from build123d import *

# Parameters (mm, degrees)
F0_R      = 19.05
F0_R_2    = 17.78
F0_R_3    = 9.525
F1_DEPTH  = 1.27
F2_DEPTH  = 151.13
F3_DEPTH  = 76.2
F5_DEPTH  = 25
F6_START  = -5.08
F6_DEPTH  = 3.302
F7_DEPTH  = 1
F8_DEPTH  = 1
F10_DEPTH = 25


with BuildPart() as f1:
    # F0 (on Top) → F1 (new body)
    with BuildSketch(Plane.XY):
        with Locations((-55.5866120592, 34.7886830568)):
            Circle(F0_R)
        with Locations((-55.5866120592, 34.7886830568)):
            Circle(F0_R_2, mode=Mode.SUBTRACT)
        with Locations((-55.5866120592, 34.7886830568)):
            Circle(F0_R_2)
        with Locations((-55.5866120592, 34.7886830568)):
            Circle(F0_R_3, mode=Mode.SUBTRACT)
        with BuildLine():
            ThreePointArc((4.7383879408, 34.7886830568), (-9.5491120592, 49.0761830568), (-23.8366120592, 34.7886830568))
            ThreePointArc((-23.8366120592, 34.7886830568), (-9.5491120592, 20.5011830568), (4.7383879408, 34.7886830568))
        make_face()
        Polygon((2.9366439238, 30.5109386121), (-7.0108694278, 21.8368289678), (-19.4966254107, 26.1145734125), (-22.0348680421, 39.0664275016), (-12.0873546906, 47.7405371459), (0.3984012923, 43.4627927011), align=None, mode=Mode.SUBTRACT)
        Polygon((-19.4966254107, 26.1145734125), (-7.0108694278, 21.8368289678), (2.9366439238, 30.5109386121), (0.3984012923, 43.4627927011), (-12.0873546906, 47.7405371459), (-22.0348680421, 39.0664275016), align=None)
    extrude(amount=-F1_DEPTH)

    # F0 (on Top) → F2 (join)
    with BuildSketch(Plane.XY):
        with Locations((-55.5866120592, 34.7886830568)):
            Circle(F0_R)
        with Locations((-55.5866120592, 34.7886830568)):
            Circle(F0_R_2, mode=Mode.SUBTRACT)
        with BuildLine():
            ThreePointArc((4.7383879408, 34.7886830568), (-9.5491120592, 49.0761830568), (-23.8366120592, 34.7886830568))
            ThreePointArc((-23.8366120592, 34.7886830568), (-9.5491120592, 20.5011830568), (4.7383879408, 34.7886830568))
        make_face()
        Polygon((2.9366439238, 30.5109386121), (-7.0108694278, 21.8368289678), (-19.4966254107, 26.1145734125), (-22.0348680421, 39.0664275016), (-12.0873546906, 47.7405371459), (0.3984012923, 43.4627927011), align=None, mode=Mode.SUBTRACT)
    extrude(amount=F2_DEPTH)



with BuildPart() as f3:
    # F0 (on Top) → F3 (new body)
    with BuildSketch(Plane.XY):
        Polygon((-36.5366120592, 53.8386830568), (-36.5366120592, 34.7886830568), (-36.5366120592, 15.7386830568), (-23.8366120592, 15.7386830568), (-23.8366120592, 34.7886830568), (-23.8366120592, 53.8386830568), align=None)
    extrude(amount=F3_DEPTH)

    # F4 (on face) → F5 (cut)
    with BuildSketch(Plane.YZ.offset(-23.8366120592)):
        Polygon((15.7386830568, 76.2), (53.8386830568, 44.2303040521), (53.8386830568, 76.2), align=None)
        Polygon((53.8386830568, 0), (53.8386830568, 9.1670642607), (15.7386830568, 41.1367602085), (15.7386830568, 0), align=None)
    extrude(amount=-F5_DEPTH, mode=Mode.SUBTRACT)

    # F4 (on face) → F6 (cut)
    with BuildSketch(Plane.YZ.offset(-23.8366120592).offset(F6_START)):
        Polygon((53.8386830568, 11.7778788393), (53.8386830568, 41.6194894735), (15.7386830568, 73.5891854213), (15.7386830568, 43.7475747872), align=None)
    extrude(amount=-F6_DEPTH, mode=Mode.SUBTRACT)


with BuildPart() as f1_1:
    add(f1.part)
    # F7 (add): a face of the model
    f7_faces = [f3.part.faces().sort_by_distance(p)[0] for p in [
        (-36.5366120592, 34.7886830568, 42.6835321303),
    ]]

    add(f3.part)  # F7 merges F3
    extrude(f7_faces, amount=F7_DEPTH)

    # F8 (add): faces of the model
    f8_faces = [f1_1.faces().sort_by_distance(p)[0] for p in [
        (-23.8366120592, 25.2636830568, 50.6759561173),
        (-23.8366120592, 44.3136830568, 34.6911081434),
    ]]
    extrude(f8_faces, amount=F8_DEPTH)

    # F9 (on face) → F10 (cut)
    with BuildSketch(Plane(origin=(0, 0, -1.27), x_dir=(1, 0, 0), z_dir=(0, 0, -1))):
        Polygon((-12.0873546906, -47.7405371459), (-5.8444766991, -45.6016649235), (-17.0611113664, -43.4034823237), align=None)
    extrude(amount=-F10_DEPTH, mode=Mode.SUBTRACT)


solid = f1_1.part
CAD build for the part. Positions are in the model's coordinates, mm. A direction names the side the tool comes from. Coordinates: 2 decimals unless noted, no trailing zeros. Order: outer loops, then holes, each group sorted by start corner. A loop starts at its lowest first (then second) coordinate and runs counter-clockwise, first axis right, second up. Notation, with made-up numbers: (70, 82.25) -> (82, 82.25) arc R24 ccw to (82, 109.25) -> close; hole circle Ø8 at (47, 39). An arc over 180 degrees is marked (long way). Answer in a Markdown table with one row per item.
1) Mould opens along X. For faces 1 (the face through (-28.917, 35, 43)), 2 (the face through (-13.166, 23.946, 74.507)), 3 (the face through (-52, 44, -1.27)) say: pulls with the +X half, pulls with the -X half, needs draft (parallel to the pull), parting line crosses it, or undercut.
Check values:
| item | result |
|---|---|
| face 1 | undercut |
| face 2 | undercut |
| face 3 | needs draft |
2) Band-saw the part on B-B (y = 33). List the corners of the cut face in (x, z).
Check values:
| item | result |
|---|---|
| outline | (-74.55, -1.27) -> (-64.94, -1.27) -> (-64.94, 0) -> (-73.28, 0) -> (-73.28, 151.13) -> (-74.55, 151.13) -> close; (-46.23, -1.27) -> (-36.62, -1.27) -> (-36.62, 26.65) -> (-23.72, 26.65) -> (-23.72, -1.27) -> (4.63, -1.27) -> (4.63, 151.13) -> (2.45, 151.13) -> (2.45, 0) -> (-20.85, 0) -> (-20.85, 151.13) -> (-23.72, 151.13) -> (-23.72, 61.72) -> (-36.62, 61.72) -> (-36.62, 151.13) -> (-37.9, 151.13) -> (-37.9, 0) -> (-46.23, 0) -> close; hole (-32.22, 29.26) -> (-28.92, 29.26) -> (-28.92, 59.11) -> (-32.22, 59.11) -> close |
3) Drill centre lines: line 1 (X direction, y = 34, z = 125); line 2 (X direction, y = 42.5, z = 66); line 3 (Y direction, x = -62, z = 8). Where is each one in solid material? Low to high.
Check values:
| item | result |
|---|---|
| line 1 | -74.62 to -73.35, -37.82 to -36.55, -23.81 to -21.04, 2.25 to 4.72 |
| line 2 | -73.01 to -71.61, -39.57 to -38.17, -21.58 to -18.1, 0.59 to 2.48 |
| line 3 | 16.85 to 18.21, 51.37 to 52.73 |
4) Band-saw the part on A-A (z = 131). Give the number of separate pieces and of enclosed holes in the cut face, and give its area (3 significant figures).
Check values:
| item | result |
|---|---|
| separate pieces | 2 |
| enclosed holes | 2 |
| area | 336 mm2 |
5) Flat gauge pins, fed straight in: P1, Ø6, axis at x = -29, z = 31, coming from the -Y side; P2, Ø11, axis at y = 45.5, z = 30, coming from the +X side; P3, Ø3, axis at x = -65.5, y = 35, coming from the +Z side. Where does each tip first touch, or does it go through?
Check values:
| item | result |
|---|---|
| P1 | y = 24.24 |
| P2 | x = 3.75 |
| P3 | z = 0 |
6) Which spindle directions (+Z, -Z, +X, -X, +Y, -Y) get a long thin tool onto all of the face, cutting with end or side? Do faces 4 (the face through (-20.75, 32.5, 74.51)), 5 (the face through (-32.219, 35, 43)), 6 (the face through (-4.3, 45.4, 151.13)). Say none if no direction does.
Check values:
| item | result |
|---|---|
| face 4 | +Z |
| face 5 | none |
| face 6 | +Z, +X, -X, +Y, -Y |
7) Band-saw the part on C-C (x = -10.5). List the corners of the cut face in (y, z).
Check values:
| item | result |
|---|---|
| outline | (20.53, -1.27) -> (44.69, -1.27) -> (44.69, 0) -> (23.03, 0) -> (23.03, 151.13) -> (20.53, 151.13) -> close; (47.2, -1.27) -> (49.04, -1.27) -> (49.04, 151.13) -> (47.2, 151.13) -> close |
